Build history of the part. All positions in model axes, mm. Give positions to 0.01 mm unless a question says otherwise; leave off trailing zeros. Write each loop counter-clockwise with the first axis right and the second up, starting at its lowest first coordinate (ties: lowest second). Pieces come first, ordered by that corner, then holes. Notation, with made-up numbers: (-17, 37.5) -> (4, 37.5) arc R5 cw to (4, 44.5) -> close; hole circle Ø11 at (80, 24). An arc over 180 degrees is marked (long way). One line per question, with ' | ' between items. Start each with the question number.
(1) Band-saw the part on B-B, the plane z = -31.5. Give the cut face in (x, y), and give its area (3 significant figures).
(2) Band-saw the part on D-D, the plane z = 13. Give the cut face in (x, y).
(3) Band-saw the part on A-A, the plane y = -53. Give the cut face in (x, z).
(4) Pin check, flat tips, straight feed: P1, Ø0.9, axis at x = 1.5, z = -82, coming from the -Y side; P2, Ø0.9, axis at x = 2, z = -79.5, coming from the +Y side. Stop position of each tip, or through.
(5) Drill centre lines: probe 1 along Y at (x, z) = (0.8, 32.5); probe 2 along Y at (x, z) = (2.5, 76.5); probe 3 along Z at (x, y) = (2.6, -55). Where is each one in solid material? Low to high. Write a range as from..to.
(6) Band-saw the part on C-C, the plane x = 0.8. Give the cut face in (y, z), and give its area (3 significant figures).
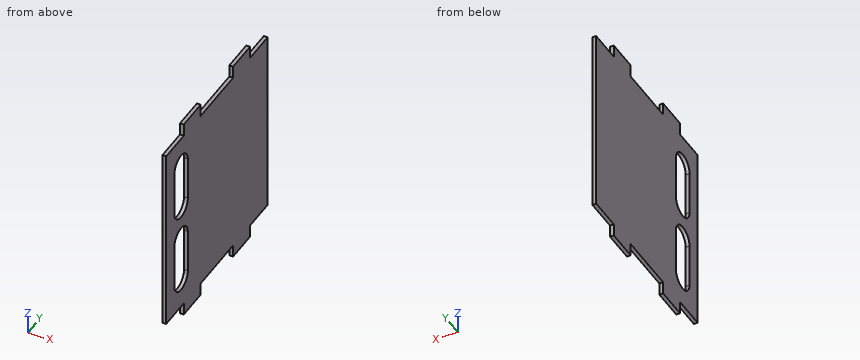
Autodesk Inventor part; units mm, degrees
ref_plane "YZ Plane" through (0, 0, 0) normal (1, 0, 0) x (0, 1, 0)
ref_plane "XZ Plane" through (0, 0, 0) normal (0, 1, 0) x (-1, 0, 0)
ref_plane "XY Plane" through (0, 0, 0) normal (0, 0, 1) x (1, 0, 0)
sketch "Sketch1" plane through (0, 0, 0) normal (1, 0, 0) x (0, 1, 0)
  line L0 (75, 75) -> (75, -75)
  line L1 (-75, -75) -> (-75, 75)
  line L2 (-75, 75) -> (75, -75) construction
  line L3 (75, 75) -> (-75, -75) construction
  line L4 (-53, 50) -> (-53, 15) construction
  line L5 (-63, 50) -> (-63, 15)
  line L6 (-43, 15) -> (-43, 50)
  arc A0 (-43, 50) -> (-63, 50) centre (-53, 50) ccw
  arc A1 (-63, 15) -> (-43, 15) centre (-53, 15) ccw
  line L7 (-53, -15) -> (-53, -50) construction
  line L8 (-43, -15) -> (-43, -50)
  line L9 (-63, -50) -> (-63, -15)
  arc A2 (-43, -15) -> (-63, -15) centre (-53, -15) ccw
  arc A3 (-63, -50) -> (-43, -50) centre (-53, -50) ccw
  line L10 (49, 75) -> (49, 85)
  line L11 (49, 85) -> (24, 85)
  line L12 (24, 85) -> (24, 75)
  line L13 (0, 0) -> (0, 108)
  line L14 (-49, 75) -> (-49, 85)
  line L15 (-49, 85) -> (-24, 85)
  line L16 (-24, 85) -> (-24, 75)
  line L17 (0, 0) -> (84, 0)
  line L18 (49, -75) -> (49, -85)
  line L19 (49, -85) -> (24, -85)
  line L20 (24, -85) -> (24, -75)
  line L21 (-49, -75) -> (-49, -85)
  line L22 (-49, -85) -> (-24, -85)
  line L23 (-24, -85) -> (-24, -75)
  line L24 (49, 75) -> (75, 75)
  line L25 (-75, 75) -> (-49, 75)
  line L26 (-24, 75) -> (24, 75)
  line L27 (75, -75) -> (49, -75)
  line L28 (24, -75) -> (-24, -75)
  line L29 (-49, -75) -> (-75, -75)
  point P0 (-53, 32.5)
  point P1 (-53, -32.5)
  dimension "d0" = 150
  dimension "d1" = 150
  dimension "d2" = 25
  dimension "d4" = 25
  dimension "d5" = 35
  dimension "d6" = 35
  dimension "d7" = 22
  dimension "d8" = 10
  dimension "d9" = 10
  dimension "d12" = 25
  dimension "d13" = 26
  dimension "d14" = 10
  dimension "d15" = 10
  dimension "d16" = 9
  dimension "d17" = 183
extrude "Extrusion1" add sketch "Sketch1" along normal blind 3
properties part number "back_part"
Results:
1) outline: (0, -75) -> (3, -75) -> (3, -63) -> (0, -63) -> close; (0, -43) -> (3, -43) -> (3, 75) -> (0, 75) -> close | area: 390 mm²
2) outline: (0, -75) -> (3, -75) -> (3, -62.8) -> (0, -62.8) -> close; (0, -43.2) -> (3, -43.2) -> (3, 75) -> (0, 75) -> close
3) outline: (0, -75) -> (3, -75) -> (3, -60) -> (0, -60) -> close; (0, -5) -> (3, -5) -> (3, 5) -> (0, 5) -> close; (0, 60) -> (3, 60) -> (3, 75) -> (0, 75) -> close
4) P1: stops at y = -49 | P2: stops at y = 49
5) probe 1: y = -75..-63, -43..75 | probe 2: y = -49..-24, 24..49 | probe 3: z = -75..-59.8, -5.2..5.2, 59.8..75
6) outline: (-75, -75) -> (-49, -75) -> (-49, -85) -> (-24, -85) -> (-24, -75) -> (24, -75) -> (24, -85) -> (49, -85) -> (49, -75) -> (75, -75) -> (75, 75) -> (49, 75) -> (49, 85) -> (24, 85) -> (24, 75) -> (-24, 75) -> (-24, 85) -> (-49, 85) -> (-49, 75) -> (-75, 75) -> close; hole (-63, -50) arc R10 ccw to (-43, -50) -> (-43, -15) arc R10 ccw to (-63, -15) -> close; hole (-63, 15) arc R10 ccw to (-43, 15) -> (-43, 50) arc R10 ccw to (-63, 50) -> close | area: 21,500 mm²
